Design review of the part built by this model. Coordinates are the model's own, in mm. Face numbers are marked on the shaded views. Give positions to 0.01 mm unless a question says otherwise; leave off trailing zeros. Order: outer loops, then holes, each group sorted by start corner. A loop starts at its lowest first (then second) coordinate and runs counter-clockwise, first axis right, second up. Notation, with made-up numbers: M 48,41 L 95,41 A20 cw 95,60 Z; hole C 27.25,-5.75 d9. An arc over 180 degrees is marked long. Answer as a JSON object with one key per item and string values.
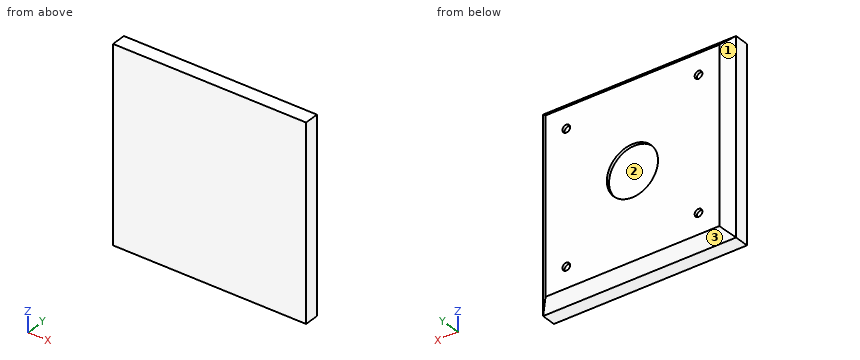
Autodesk Inventor part; units mm, degrees
ref_plane "YZ Plane" through (0, 0, 0) normal (1, 0, 0) x (0, 1, 0)
ref_plane "XZ Plane" through (0, 0, 0) normal (0, 1, 0) x (-1, 0, 0)
ref_plane "XY Plane" through (0, 0, 0) normal (0, 0, 1) x (1, 0, 0)
sketch "Skizze1" plane through (0, 0, 0) normal (0, 1, 0) x (-1, 0, 0)
  line L0 (-100, 100) -> (100, 100)
  line L1 (100, 100) -> (100, -100)
  line L2 (100, -100) -> (-100, -100)
  line L3 (-100, -100) -> (-100, 100)
  line L4 (-100, 100) -> (100, -100) construction
  line L5 (100, 100) -> (-100, -100) construction
  point P0 (0, 0)
  dimension "d0" = 200
  dimension "d1" = 200
extrude "Extrusion1" add sketch "Skizze1" along normal blind 25
chamfer "Fasen1" distance 10 angle 45 4 edges at (100, 25, 0) (0, 25, 100) (0, 25, -100) (-100, 25, 0)
sketch "Skizze2" plane through (0, 25, 0) normal (0, 1, 0) x (1, 0, 0)
  point P0 (0, 0)
  point P1 (0, 0)
hole "Bohrung1" at (0, 25, 0) direction (0, -1, 0) diameter 53 depth 3
sketch "Skizze3" plane through (0, 25, 0) normal (0, 1, 0) x (1, 0, 0)
  line L0 (90, -90) -> (-90, -90)
  line L1 (0, -90) -> (0, 90) construction
  line L2 (-90, 90) -> (90, 90)
  line L3 (-90, -90) -> (-90, 90)
  line L4 (-90, 0) -> (90.2684, 0) construction
  point P0 (0, 0)
  point P1 (-68.5, -68.5)
  point P2 (68.5, -68.5)
  point P3 (68.5, 68.5)
  point P4 (-68.5, 68.5)
  point P5 (0.1342, 0)
  dimension "d21" = 68.5
  dimension "d22" = 68.5
  dimension "d23" = 137
  dimension "d24" = 68.5
  dimension "d25" = 68.5
hole "Bohrung2" at (-68.5, 25, 68.5) at (68.5, 25, 68.5) at (68.5, 25, -68.5) at (-68.5, 25, -68.5) direction (0, -1, 0) diameter 8 depth 3
properties part number "wooden support" material "Holz (Ahorn)"
(1) We need section D-D (z = 68.5). Write out the cut boundary in (x, y), plus the area to 3 significant figures.
Checked values:
{"outline": "M -100,0 L 100,0 L 100,15 L 90,25 L 72.5,25 L 72.5,22 L 64.5,22 L 64.5,25 L -64.5,25 L -64.5,22 L -72.5,22 L -72.5,25 L -90,25 L -100,15 Z", "area": "4,850 mm^2"}
(2) We need section B-B (x = 0). Write out the cut boundary in (y, z).
Checked values:
{"outline": "M 0,-100 L 15,-100 L 25,-90 L 25,-26.5 L 22,-26.5 L 22,26.5 L 25,26.5 L 25,90 L 15,100 L 0,100 Z"}
(3) We need section A-A (z = 0). Write out the cut boundary in (x, y).
Checked values:
{"outline": "M -100,0 L 100,0 L 100,15 L 90,25 L 26.5,25 L 26.5,22 L -26.5,22 L -26.5,25 L -90,25 L -100,15 Z"}
(4) Insertion check: pin 1 (12 mm diameter, centred on x = 60.5, y = 21.5, fed in from -Z); pin 2 (4 mm diameter, centred on x = 68.5, z = -69.5, fed in from +Y); pin 3 (4 mm diameter, centred on y = 21, z = 71, fed in from -X). Each pin has a flat end and moves straight along its axis. Give the tip position at first contact, or say it passes through.
Checked values:
{"pin 1": "stops at z = -99.5", "pin 2": "stops at y = 22", "pin 3": "stops at x = -96"}
(5) We need section C-C (y = 18.5). Write out the cut boundary in (x, z).
Checked values:
{"outline": "M -96.5,-96.5 L 96.5,-96.5 L 96.5,96.5 L -96.5,96.5 Z"}
(6) Draft analysis for pull direction Z (two halves, no side actions). For the marked faces 1, 2 and 3, state which applies: +Z half, -Z half, draft (parallel to the pull), parting line (faces both ways), or undercut.
Checked values:
{"face 1": "draft", "face 2": "undercut", "face 3": "-Z half"}
(7) To check wall thickness, follow L1, parallel to X at y = 22.85, z = 68.5; L2, parallel to Z at x = -68.5, y = 23.55; L3, parallel to X at y = 23.5, z = 68.5. State the ranges of each line that lie inside material, in increasing order. Write a range as from..to.
Checked values:
{"L1": "x = -92.15..-72.5, -64.5..64.5, 72.5..92.15", "L2": "z = -91.45..-72.5, -64.5..64.5, 72.5..91.45", "L3": "x = -91.5..-72.5, -64.5..64.5, 72.5..91.5"}
